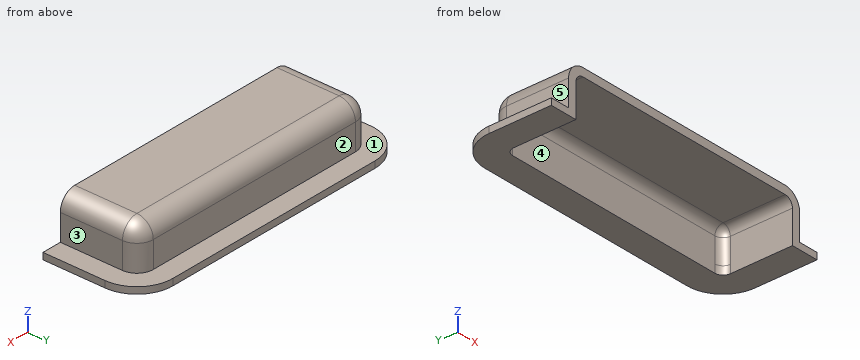
```python
from build123d import *

# Parameters (mm, degrees)
F1_DEPTH = 2
F3_DEPTH = 15
F4_R     = 5
F5_T     = -2.5
F7_DEPTH = 25


with BuildPart() as f1:
    # F0 (on Top) → F1 (new body)
    with BuildSketch(Plane.XY):
        with BuildLine():
            Line((-46, 19), (-46, 0))
            Line((-46, 0), (-40, 0))
            Line((-40, 0), (-40, 19))
            ThreePointArc((-40, 19), (-38.5355339059, 22.5355339059), (-35, 24))
            Line((-35, 24), (35, 24))
            ThreePointArc((35, 24), (38.5355339059, 22.5355339059), (40, 19))
            Line((40, 19), (40, 0))
            Line((40, 0), (46, 0))
            Line((46, 0), (46, 19))
            ThreePointArc((46, 19), (42.7781745931, 26.7781745931), (35, 30))
            Line((35, 30), (-35, 30))
            ThreePointArc((-35, 30), (-42.7781745931, 26.7781745931), (-46, 19))
        make_face()
    extrude(amount=F1_DEPTH)

    # F2 (on Top) → F3 (join)
    with BuildSketch(Plane.XY):
        with BuildLine():
            Line((-40, 0), (40, 0))
            Line((40, 0), (40, 19))
            ThreePointArc((40, 19), (38.5355339059, 22.5355339059), (35, 24))
            Line((35, 24), (-35, 24))
            ThreePointArc((-35, 24), (-38.5355339059, 22.5355339059), (-40, 19))
            Line((-40, 19), (-40, 0))
        make_face()
    extrude(amount=F3_DEPTH)

    # F4
    f4_edges = [f1.edges().sort_by_distance(p)[0] for p in [
        (-40, 9.5, 15),
    ]]
    fillet(f4_edges, radius=F4_R)

    # F5
    f5_openings = [f1.faces().sort_by_distance(p)[0] for p in [
        (0, 0, 7.31497),
    ]]
    offset(amount=F5_T, openings=f5_openings)

    # F6 (on face) → F7 (cut)
    with BuildSketch(Plane.XY.offset(2.5)):
        with BuildLine():
            ThreePointArc((37.5, 19), (36.767766953, 20.767766953), (35, 21.5))
            Line((35, 21.5), (-35, 21.5))
            ThreePointArc((-35, 21.5), (-36.767766953, 20.767766953), (-37.5, 19))
            Line((-37.5, 19), (-37.5, 0))
            Line((-37.5, 0), (37.5, 0))
            Line((37.5, 0), (37.5, 19))
        make_face()
    extrude(amount=-F7_DEPTH, mode=Mode.SUBTRACT)


solid = f1.part
```
Input: part model. Units: mm. Frame: model coordinates. Face numbers are marked on the shaded views. A direction names the side the tool comes from. Coordinates: 2 decimals unless noted, no trailing zeros. Order: outer loops, then holes, each group sorted by start corner. A loop starts at its lowest first (then second) coordinate and runs counter-clockwise, first axis right, second up. Notation, with made-up numbers: (-1.75, 61) - (33.25, 61) arc R33 cw to (33.25, 94) - close; hole circle Ø2 at (48.25, 15.5). An arc over 180 degrees is marked (long way). Put each result on its own line as item: value.
1. Cut plane A-A on x = -13.5. Return the cut outline in (y, z).
Report:
outline: (0, 12.5) - (19, 12.5) arc R2.5 cw to (21.5, 10) - (21.5, 0) - (30, 0) - (30, 2) - (24, 2) - (24, 10) arc R5 ccw to (19, 15) - (0, 15) - close
2. Reachability of the marked faces 1, 2, 3, 4 and 5 from +Z, -Z, +X, -X, +Y, -Y: full face, straight path, thin tool, end or side. Return the list, or none.
Report:
face 1: +Z, +Y
face 2: +Z, +X, -X, +Y
face 3: +Z, +X, +Y, -Y
face 4: -Z, -Y
face 5: +Z, -X, +Y, -Y
3. Cut plane B-B on z = 8.25. Return the cut outline in (x, y), then the cut area to 3 significant figures.
Report:
outline: (-40, 0) - (-37.5, 0) - (-37.5, 19) arc R2.5 cw to (-35, 21.5) - (35, 21.5) arc R2.5 cw to (37.5, 19) - (37.5, 0) - (40, 0) - (40, 19) arc R5 ccw to (35, 24) - (-35, 24) arc R5 ccw to (-40, 19) - close
area: 299 mm2
4. Cut plane C-C on y = 3.75. Return the cut outline in (x, z).
Report:
outline: (-46, 0) - (-37.5, 0) - (-37.5, 10) arc R2.5 cw to (-35, 12.5) - (35, 12.5) arc R2.5 cw to (37.5, 10) - (37.5, 0) - (46, 0) - (46, 2) - (40, 2) - (40, 10) arc R5 ccw to (35, 15) - (-35, 15) arc R5 ccw to (-40, 10) - (-40, 2) - (-46, 2) - close
5. Cut plane D-D on z = 14. Return the cut outline in (x, y).
Report:
outline: (-38, 0) - (38, 0) - (38, 19) arc R3 ccw to (35, 22) - (-35, 22) arc R3 ccw to (-38, 19) - close
6. Line query: line 1 along X through (y, z) = (8, 7.5); line 2 along Y through (x, z) = (19.5, 5.5); line 3 along Z through (x, y) = (-17.5, 13.5). Output: solid intervals per line, ascending.
Report:
line 1: x = -40 to -37.5, 37.5 to 40
line 2: y = 21.5 to 24
line 3: z = 12.5 to 15
7. Contact query for flat-ended pins moving along their axis: pin 1 Ø8 at (x, z) = (-11, 12.5) entering from +Y; pin 2 Ø5 at (x, z) = (-4, 3.5) entering from -Y; pin 3 Ø2.5 at (y, z) = (6, 4.5) entering from +X; pin 4 Ø12 at (x, y) = (7, 18.5) entering from -Z. Output: stop coordinate, or through.
Report:
pin 1: stops at y = 24
pin 2: stops at y = 21.5
pin 3: stops at x = 40
pin 4: stops at z = 0
